from build123d import *

# Parameters (mm, degrees)
F3_R = 2


with BuildPart() as f2:
    # F2: sweep along a path in F1
    with BuildLine(Plane.XY) as f2_path:
        Line((0, 0), (920, 0))
    # F0 (on Right) → F2 (sweep)
    with BuildSketch(Plane.YZ):
        Polygon((38, -2), (38, -25), (40, -25), (40, 0), (0, 0), (0, -100), (27, -100), (27, -126), (29, -126), (29, -98), (2, -98), (2, -2), align=None)
    sweep(path=f2_path.line)

    # F3
    f3_edges = [f2.edges().sort_by_distance(p)[0] for p in [
        (460, 40, 0),
        (460, 0, 0),
        (460, 29, -98),
        (460, 2, -98),
        (460, 2, -2),
        (460, 38, -2),
        (460, 0, -100),
        (460, 27, -100),
    ]]
    fillet(f3_edges, radius=F3_R)


solid = f2.part
Part model, mm, in its own coordinate system. A direction names the side the tool comes from. Give positions to 0.01 mm unless a question says otherwise; leave off trailing zeros. Loops run counter-clockwise (first coordinate to the right, second up) from the corner with the lowest first, then second, coordinate; pieces in that order, holes last. Notation, with made-up numbers: (-22.75, -8) -> (-3.75, -8) arc R34 cw to (-3.75, 30) -> close; hole circle Ø11 at (5, 44.25). An arc over 180 degrees is marked (long way). Write each question's results on one line, items separated by ' | '. Start each with the question number.
Q1. Band-saw the part on B-B on z = -82. List the corners of the cut face in (x, y).
Q2. Pull direction Z, two halves, no side cores. Call faces 6 (the face through (466, 38, -14)), 7 (the face through (466, 2, -51)), 8 (the face through (466, 13, -100)): +Z half, -Z half, draft (parallel to the pull), parting line (faces both ways), or undercut.
Q3. Wall check: L1, parallel to Z at x = 579, y = 17.5; L2, parallel to Y at x = 259, z = -22; L3, parallel to Y at x = 735.5, z = -109.5. Give the ranges that are in metal, low to high.
Q4. Which spindle directions (+Z, -Z, +X, -X, +Y, -Y) get a long thin tool onto all of the face, cutting with end or side? Do faces 1 (the face through (466, 20, -2)), 2 (the face through (466, 16, -98)), 3 (the face through (466, 27, -114)), 4 (the face through (466, 29, -113)), 5 (the face through (466, 0, -49)). Say none if no direction does.
Q5. Band-saw the part on A-A on x = 474. List the corners of the cut face in (y, z), plus the area to 3 significant figures.
Q6. Pin check, flat tips, straight feed: P1, Ø3, axis at x = 562, z = -71.5, coming from the +Y side; P2, Ø8, axis at x = 432.5, z = -111.5, coming from the +Y side; P3, Ø11.5, axis at x = 669, y = 8, coming from the -Z side. Stop position of each tip, or through.
Results are:
1) outline: (0, 0) -> (920, 0) -> (920, 2) -> (0, 2) -> close
2) face 6: draft | face 7: undercut | face 8: -Z half
3) L1: z = -100 to -98, -2 to 0 | L2: y = 0 to 2, 38 to 40 | L3: y = 27 to 29
4) face 1: +X, -X | face 2: +X, -X, +Y | face 3: -Z, +X, -X, -Y | face 4: -Z, +X, -X, +Y | face 5: +Z, -Z, +X, -X, -Y
5) outline: (0, -98) arc R2 ccw to (2, -100) -> (25, -100) arc R2 cw to (27, -102) -> (27, -126) -> (29, -126) -> (29, -100) arc R2 ccw to (27, -98) -> (4, -98) arc R2 cw to (2, -96) -> (2, -4) arc R2 cw to (4, -2) -> (36, -2) arc R2 cw to (38, -4) -> (38, -25) -> (40, -25) -> (40, -2) arc R2 ccw to (38, 0) -> (2, 0) arc R2 ccw to (0, -2) -> close | area: 428 mm²
6) P1: stops at y = 2 | P2: stops at y = 29 | P3: stops at z = -100
